Verification items for the finished model (mm, model axes). Face numbers are marked on the shaded views. A direction names the side the tool comes from. Round coordinates to 2 decimals unless told otherwise and drop trailing zeros. Order: outer loops, then holes, each group sorted by start corner. A loop starts at its lowest first (then second) coordinate and runs counter-clockwise, first axis right, second up. Notation, with made-up numbers: M -37.5,-29.75 L 6.5,-29.75 A26 ccw 6.5,-2.75 Z; hole C 56,69.25 d7. An arc over 180 degrees is marked long. Use one line per item in the form item = value. Start each with the question number.
Item 1: Cross-section at B-B on x = -22. Enter the section's corners in (y, z).
Item 2: Go/stop test with flat-tipped pins: pin 1 Ø1 at (x, y) = (-13.5, 11) entering from +Z; pin 2 Ø3 at (x, y) = (-20, 15) entering from -Z; pin 3 Ø2 at (x, z) = (-3.5, -8) entering from +Y; pin 4 Ø1.8 at (x, y) = (-20.5, 13.5) entering from +Z. Record where each tip stops, or that it passes through.
Item 3: Cross-section at A-A on y = 15. Enter the section's corners in (x, z).
Item 4: Cross-section at C-C on z = -6.5. Enter the section's corners in (x, y).
Item 5: Cross-section at D-D on y = 7. Enter the section's corners in (x, z).
Item 6: Release check for a two-part mould opening along Y. For the marked faces 1, 2, 3 and 4 record: +Y half, -Y half, draft (parallel to the pull), parting line (faces both ways), or undercut.
Item 7: Tool access check on the marked faces 5, 6 and 7. Record the directions out of +Z, -Z, +X, -X, +Y, -Y that give a thin tool (end or side, any length) a straight path to the whole face; none if there is none.
Item 8: Thickness scan on probe 1 along Y at (x, z) = (-20, -16.15); probe 2 along Y at (x, z) = (-20, -3.7); probe 3 along Z at (x, y) = (-20, 7.75). Record the ranges inside material, lowest first. Write a range as [from, to].
Autodesk Inventor part; units mm, degrees
ref_plane "YZ Plane" through (0, 0, 0) normal (1, 0, 0) x (0, 1, 0)
ref_plane "XZ Plane" through (0, 0, 0) normal (0, 1, 0) x (-1, 0, 0)
ref_plane "XY Plane" through (0, 0, 0) normal (0, 0, 1) x (1, 0, 0)
sketch "Sketch1" plane through (0, 0, 0) normal (0, 1, 0) x (-1, 0, 0)
  line L0 (0, 0) -> (25, 0)
  line L1 (25, 0) -> (25, -17)
  line L2 (25, -17) -> (0, -17)
  line L3 (0, -17) -> (0, 0)
  dimension "d0" = 17
  dimension "d1" = 25
extrude "Extrusion1" add sketch "Sketch1" along normal blind 20
sketch "Sketch2" plane through (0, 20, 0) normal (0, 1, 0) x (1, 0, 0)
  circle A0 centre (-8.5, 8.5) radius 5
  line L0 (-25, 0) -> (0, 0)
  line L1 (0, 0) -> (0, 17)
  dimension "d4" = 10
  dimension "d5" = 8.5
  dimension "d6" = 8.5
extrude "Extrusion2" cut sketch "Sketch2" against normal through all
sketch "Sketch3" plane through (0, 20, 0) normal (0, 1, 0) x (1, 0, 0)
  circle A0 centre (-8.5, 8.5) radius 6.5
  line L0 (-25, 0) -> (0, 0)
  line L1 (0, 0) -> (0, 17)
  dimension "d9" = 13
  dimension "d10" = 8.5
  dimension "d11" = 8.5
extrude "Extrusion3" cut sketch "Sketch3" against normal blind 10
sketch "Sketch4" plane through (0, 20, 0) normal (0, 1, 0) x (1, 0, 0)
  line L0 (-25, 17) -> (-25, 0)
  line L1 (-25, 7.5) -> (-12, 7.5)
  line L2 (-12, 7.5) -> (-12, 9.5)
  line L3 (-12, 9.5) -> (-25, 9.5)
  line L4 (-25, 9.5) -> (-25, 7.5)
  line L5 (-25, 0) -> (0, 0)
  dimension "d14" = 2
  dimension "d15" = 7.5
  dimension "d16" = 13
extrude "Extrusion4" cut sketch "Sketch4" against normal through all
sketch "Sketch5" plane through (0, 20, 0) normal (0, 1, 0) x (1, 0, 0)
  line L0 (-23, 0) -> (-17, 0)
  line L1 (-17, 0) -> (-17, 2.5)
  line L2 (-17, 2.5) -> (-23, 2.5)
  line L3 (-23, 2.5) -> (-23, 0)
  line L4 (-25, 7.5) -> (-25, 0)
  line L5 (-25, 0) -> (0, 0)
  dimension "d19" = 6
  dimension "d20" = 2.5
  dimension "d21" = 2
extrude "Extrusion5" cut sketch "Sketch5" against normal through all
sketch "Sketch6" plane through (0, 0, -17) normal (0, 0, -1) x (-1, 0, 0)
  circle A0 centre (20, 15) radius 1.6
  circle A1 centre (20, 5) radius 1.6
  line L0 (25, 0) -> (25, 20)
  line L1 (0, 20) -> (25, 20)
  line L2 (0, 0) -> (25, 0)
  dimension "d24" = 3.2
  dimension "d25" = 3.2
  dimension "d26" = 5
  dimension "d27" = 5
  dimension "d28" = 5
  dimension "d29" = 5
extrude "Extrusion6" cut sketch "Sketch6" against normal through all
sketch "Sketch7" plane through (0, 0, -17) normal (0, 0, -1) x (-1, 0, 0)
  circle A0 centre (20, 5) radius 2.9
  circle A1 centre (20, 15) radius 2.9
  line L0 (25, 0) -> (25, 20)
  line L1 (0, 0) -> (25, 0)
  line L2 (0, 20) -> (25, 20)
  dimension "d32" = 5.8
  dimension "d33" = 5.8
  dimension "d34" = 5
  dimension "d35" = 5
  dimension "d36" = 5
  dimension "d37" = 5
extrude "Extrusion7" cut sketch "Sketch7" against normal blind 3
fillet "Fillet1" radius 2 3 edges at (0, 10, -17) (0, 10, 0) (-25, 10, -17)
properties part number "ACCROCHE SUR ACIER"
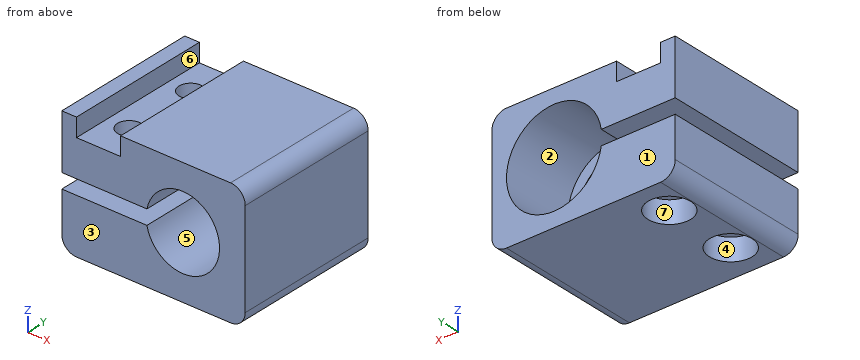
Output values:
q1.outline = M 0,-17 L 2.9,-17 L 2.9,-14 L 7.1,-14 L 7.1,-17 L 12.9,-17 L 12.9,-14 L 17.1,-14 L 17.1,-17 L 20,-17 L 20,-9.5 L 0,-9.5 Z; M 0,-7.5 L 20,-7.5 L 20,-2.5 L 0,-2.5 Z
q2.pin_1 = 0
q2.pin_2 = through
q2.pin_3 = 10
q2.pin_4 = -2.5
q3.outline = M -25,-15 A2 ccw -23,-17 L -22.9,-17 L -22.9,-14 L -21.6,-14 L -21.6,-9.5 L -25,-9.5 Z; M -25,-7.5 L -21.6,-7.5 L -21.6,-2.5 L -23,-2.5 L -23,0 L -25,0 Z; M -18.4,-14 L -17.1,-14 L -17.1,-17 L -2,-17 A2 ccw 0,-15 L 0,-2 A2 ccw -2,0 L -17,0 L -17,-2.5 L -18.4,-2.5 L -18.4,-7.5 L -14.92,-7.5 A6.5 cw long -14.92,-9.5 L -18.4,-9.5 Z
q4.outline = M -25,0 L -13.08,0 L -13.08,10 L -14.68,10 L -14.68,20 L -25,20 Z; M -3.92,0 L 0,0 L 0,20 L -2.32,20 L -2.32,10 L -3.92,10 Z; hole C -20,5 d3.2; hole C -20,15 d3.2
q5.outline = M -25,-15 A2 ccw -23,-17 L -22.1,-17 L -22.1,-14 L -17.9,-14 L -17.9,-17 L -2,-17 A2 ccw 0,-15 L 0,-2 A2 ccw -2,0 L -17,0 L -17,-2.5 L -23,-2.5 L -23,0 L -25,0 L -25,-7.5 L -13.4,-7.5 A5 cw long -13.4,-9.5 L -25,-9.5 Z
q6.face_1 = +Y half
q6.face_2 = draft
q6.face_3 = -Y half
q6.face_4 = undercut
q7.face_5 = +Y, -Y
q7.face_6 = +Z, +Y, -Y
q7.face_7 = -Z
q8.probe_1 = [0, 2.1], [7.9, 12.1], [17.9, 20]
q8.probe_2 = [0, 3.4], [6.6, 13.4], [16.6, 20]
q8.probe_3 = [-14, -9.5], [-7.5, -2.5]
